Design review of the part built by this model. Coordinates are the model's own, in mm. Coordinates: 2 decimals unless noted, no trailing zeros. Loops run counter-clockwise (first coordinate to the right, second up) from the corner with the lowest first, then second, coordinate; pieces in that order, holes last. Notation, with made-up numbers: (50, -10) - (72, -10) arc R13 cw to (72, -5) - close; hole circle Ø10 at (-16, -23.75). An arc over 180 degrees is marked (long way). Answer in a Markdown table with one row per item. Add a question column.
(1) The part is to be moulded in two halves that separate along Z. For faces 1 (the face through (33.88, 2.46, 6.07)), 2 (the face through (19, 5, 16)), 3 (the face through (19, 2, 0)), 4 (the face through (33.203, 2.465, 26.885)), say which applies: released by +Z, released by -Z, zero draft, split by the parting line, or undercut.
(2) To check wall thickness, follow L1, parallel to X at y = 2.2, z = 6.35; L2, parallel to X at y = 2.95, z = 28; L3, parallel to Z at x = 6.5, y = 0.55. State the ranges of each line that lie inside material, in increasing order. Write a range as [from, to].
(3) Clearance check with flat-ended pins moving along their axes: pin 1 (4 mm diameter, centred on x = 6.35, z = 6.35, fed in from -Y); pin 2 (10 mm diameter, centred on x = 32, z = 26, fed in from -Y). State where each tip first meets the part, or that it passes through.
(4) We need section A-A, the plane x = 6.35. Write out the cut boundary in (y, z).
(5) We need section B-B, the plane z = 6.35. Write out the cut boundary in (x, y), plus the area to 3 significant figures.
from build123d import *

# Parameters (mm, degrees)
SKETCH1_W           = 38.1
SKETCH1_H           = 32.97
SKETCH1_R           = 2.15
BOSS_EXTRUDE1_DEPTH = 5
FILLET1_R           = 5
FILLET2_R           = 1


with BuildPart() as part:
    # Sketch1 → Boss-Extrude1 (new body)
    with BuildSketch(Plane(origin=(0, 0, 0), x_dir=(1, 0, 0), z_dir=(0, 1, 0))):
        with Locations((19.05, -16.485)):
            Rectangle(SKETCH1_W, SKETCH1_H)
        with Locations(Location((6.35, -6.35, 0), (0, 0, 270))):
            Circle(SKETCH1_R, mode=Mode.SUBTRACT)
        with Locations(Location((31.75, -6.35, 0), (0, 0, 270))):
            Circle(SKETCH1_R, mode=Mode.SUBTRACT)
        with Locations(Location((31.75, -28.47, 0), (0, 0, 270))):
            Circle(SKETCH1_R, mode=Mode.SUBTRACT)
        with Locations(Location((6.35, -28.47, 0), (0, 0, 270))):
            Circle(SKETCH1_R, mode=Mode.SUBTRACT)
    extrude(amount=BOSS_EXTRUDE1_DEPTH)

    # Fillet1
    fillet1_edges = [part.edges().sort_by_distance(p)[0] for p in [
        (0, 2.5, 0),
        (38.1, 2.5, 0),
        (38.1, 2.5, 32.97),
        (0, 2.5, 32.97),
    ]]
    fillet(fillet1_edges, radius=FILLET1_R)

    # Fillet2
    fillet2_edges = [part.edges().sort_by_distance(p)[0] for p in [
        (0, 0, 16.485),
        (0, 5, 16.485),
        (19.05, 0, 0),
        (38.1, 0, 16.485),
        (19.05, 0, 32.97),
        (1.464466094, 0, 31.505533906),
        (36.635533906, 0, 31.505533906),
        (36.635533906, 0, 1.464466094),
        (1.464466094, 0, 1.464466094),
        (19.05, 5, 0),
        (19.05, 5, 32.97),
        (38.1, 5, 16.485),
        (1.464466094, 5, 31.505533906),
        (36.635533906, 5, 31.505533906),
        (36.635533906, 5, 1.464466094),
        (1.464466094, 5, 1.464466094),
    ]]
    fillet(fillet2_edges, radius=FILLET2_R)


solid = part.part
Responses:
| question | item | result |
|---|---|---|
| 1 | face 1 | undercut |
| 1 | face 2 | zero draft |
| 1 | face 3 | released by -Z |
| 1 | face 4 | undercut |
| 2 | L1 | x = [0, 4.2], [8.5, 29.6], [33.9, 38.1] |
| 2 | L2 | x = [0, 4.25], [8.45, 29.65], [33.85, 38.1] |
| 2 | L3 | z = [0.11, 4.21], [8.49, 26.33], [30.61, 32.86] |
| 3 | pin 1 | passes through |
| 3 | pin 2 | stops at y = 0 |
| 4 | outline | (0, 1) arc R1 ccw to (1, 0) - (4, 0) arc R1 ccw to (5, 1) - (5, 4.2) - (0, 4.2) - close; (0, 8.5) - (5, 8.5) - (5, 26.32) - (0, 26.32) - close; (0, 30.62) - (5, 30.62) - (5, 31.97) arc R1 ccw to (4, 32.97) - (1, 32.97) arc R1 ccw to (0, 31.97) - close |
| 5 | outline | (0, 1) arc R1 ccw to (1, 0) - (4.2, 0) - (4.2, 5) - (1, 5) arc R1 ccw to (0, 4) - close; (8.5, 0) - (29.6, 0) - (29.6, 5) - (8.5, 5) - close; (33.9, 0) - (37.1, 0) arc R1 ccw to (38.1, 1) - (38.1, 4) arc R1 ccw to (37.1, 5) - (33.9, 5) - close |
| 5 | area | 147 mm2 |
